from build123d import *

# Parameters (mm, degrees)
SKIZZE1_R                       = 6.5
AUFSATZ_LINEAR_AUSTRAGEN1_DEPTH = 2
SKIZZE2_R                       = 5
AUFSATZ_LINEAR_AUSTRAGEN2_DEPTH = 1
SKIZZE3_R                       = 6.5
AUFSATZ_LINEAR_AUSTRAGEN3_DEPTH = 2
DURCHGANGSLOCH_F_R_M51_D        = 5.5


with BuildPart() as part:
    # Skizze1 → Aufsatz-Linear austragen1 (new body)
    with BuildSketch(Plane(origin=(0, 0, 0), x_dir=(1, 0, 0), z_dir=(0, 1, 0))):
        with Locations(Location((0, 0, 0), (0, 0, 270))):
            Circle(SKIZZE1_R)
    extrude(amount=AUFSATZ_LINEAR_AUSTRAGEN1_DEPTH)

    # Skizze2 → Aufsatz-Linear austragen2 (add)
    with BuildSketch(Plane(origin=(0, 2, 0), x_dir=(1, 0, 0), z_dir=(0, 1, 0))):
        with Locations(Location((0, 0, 0), (0, 0, 270))):
            Circle(SKIZZE2_R)
    aufsatz_linear_austragen2 = extrude(amount=AUFSATZ_LINEAR_AUSTRAGEN2_DEPTH)

    # Spiegeln3: Aufsatz-Linear austragen2 across plane
    add(aufsatz_linear_austragen2.mirror(Plane.ZX.offset(3)))

    # Skizze3 → Aufsatz-Linear austragen3 (add)
    with BuildSketch(Plane(origin=(0, 4, 0), x_dir=(1, 0, 0), z_dir=(0, 1, 0))):
        with Locations(Location((0, 0, 0), (0, 0, 270))):
            Circle(SKIZZE3_R)
    extrude(amount=AUFSATZ_LINEAR_AUSTRAGEN3_DEPTH)

    # Durchgangsloch für M51 (through all)
    with Locations(Plane(origin=(0, 6, 0), x_dir=(1, 0, 0), z_dir=(0, 1, 0))):
        with Locations((0, 0)):
            Hole(DURCHGANGSLOCH_F_R_M51_D / 2)


solid = part.part
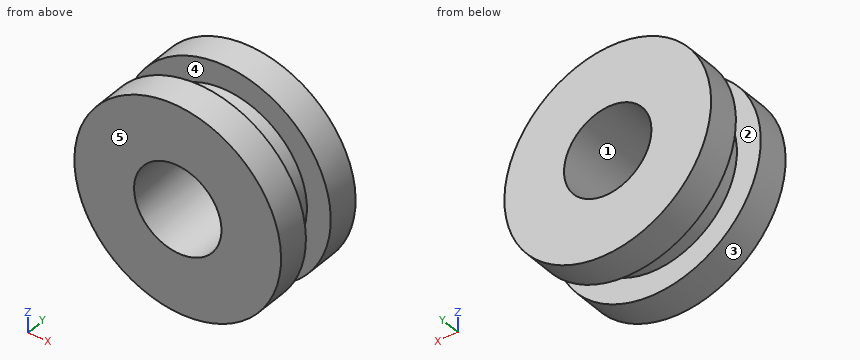
Geometry: final body of the model. Coordinates: model frame, mm. Face numbers are marked on the shaded views. A direction names the side the tool comes from. Coordinates: 2 decimals unless noted, no trailing zeros. Order: outer loops, then holes, each group sorted by start corner. A loop starts at its lowest first (then second) coordinate and runs counter-clockwise, first axis right, second up.
1) Set-up query: the marked faces 4 and 5. Return all of +Z, -Z, +X, -X, +Y, -Y with unobstructed straight access to the full face (end or side cutting, diameter ignored); none if empty.
Result sheet:
face 4: none
face 5: +Z, -Z, +X, -X, -Y
2) Section A-A (z = 0). Return loops of the section in (x, y).
Result sheet:
outline: (-6.5, 0) - (-2.75, 0) - (-2.75, 6) - (-6.5, 6) - (-6.5, 4) - (-5, 4) - (-5, 2) - (-6.5, 2) - close; (2.75, 0) - (6.5, 0) - (6.5, 2) - (5, 2) - (5, 4) - (6.5, 4) - (6.5, 6) - (2.75, 6) - close
3) Section D-D (z = 3.25). Return loops of the section in (x, y), then the cut area to 3 significant figures.
Result sheet:
outline: (-5.63, 0) - (5.63, 0) - (5.63, 2) - (3.8, 2) - (3.8, 4) - (5.63, 4) - (5.63, 6) - (-5.63, 6) - (-5.63, 4) - (-3.8, 4) - (-3.8, 2) - (-5.63, 2) - close
area: 60.2 mm2
4) First-contact query: P1, Ø1.5, axis at y = 5, z = -1.5, coming from the +X side. Flat tip, straight axial feed; report the tip coordinate or a pass-through.
Result sheet:
P1: stops at x = 6.46
5) Section B-B (x = 0). Return loops of the section in (y, z), then the cut area to 3 significant figures.
Result sheet:
outline: (0, -6.5) - (2, -6.5) - (2, -5) - (4, -5) - (4, -6.5) - (6, -6.5) - (6, -2.75) - (0, -2.75) - close; (0, 2.75) - (6, 2.75) - (6, 6.5) - (4, 6.5) - (4, 5) - (2, 5) - (2, 6.5) - (0, 6.5) - close
area: 39.0 mm2
6) Section C-C (y = 2.6). Return loops of the section in (x, z).
Result sheet:
outline: circle Ø10 at (0, 0); hole circle Ø5.5 at (0, 0)
7) Ray query, probe 1 along Y at (x, z) = (3.25, 4); probe 2 along X at (y, z) = (4.25, 1); probe 3 along Z at (x, y) = (0.5, 0.45). Return the intervals inside material, ascending.
Result sheet:
probe 1: y = 0 to 2, 4 to 6
probe 2: x = -6.42 to -2.56, 2.56 to 6.42
probe 3: z = -6.48 to -2.7, 2.7 to 6.48
8) Draft query along Z for the marked faces 1, 2 and 3. Return one class per face: released by +Z, released by -Z, zero draft, split by the parting line, or undercut.
Result sheet:
face 1: undercut
face 2: zero draft
face 3: split by the parting line
